from build123d import *

# Parameters (mm, degrees)
SKETCH_1_W      = 30
SKETCH_1_H      = 2
EXTRUDE_2_DEPTH = 2


with BuildPart() as part:
    # 草图1 → 凸台-拉伸2 (new body)
    with BuildSketch(Plane.XY):
        Polygon((-8, 49), (-8, 45), (2, 45), (2, 33.89311496), (2, -33.9722289), (2, -44.34252785), (-8, -44.34252785), (-8, -48.34252785), (-10, -48.34252785), (-10, -68.34252785), (-8, -68.34252785), (-8, -88.34252785), (-10, -88.34252785), (-10, -108.34252785), (-8, -108.34252785), (-8, -128.34252785), (-10, -128.34252785), (-10, -144), (-8, -144), (27, -144), (29, -144), (29, -128.34252785), (27, -128.34252785), (27, -108.34252785), (29, -108.34252785), (29, -88.34252785), (27, -88.34252785), (27, -68.34252785), (29, -68.34252785), (29, -48.34252785), (27, -48.34252785), (27, -28.34252785), (29, -28.34252785), (29, -8.34252785), (27, -8.34252785), (27, 11.65747215), (29, 11.65747215), (29, 31.65747215), (27, 31.65747215), (27, 51.65747215), (29, 51.65747215), (29, 59), (-10, 59), (-10, 49), align=None)
        Polygon((9.5, -54.22154055), (24.5, -54.22154055), (24.5, -56.22154055), (-5.5, -56.22154055), (-5.5, -54.22154055), align=None, mode=Mode.SUBTRACT)
        with Locations((9.5, -95.22154055)):
            Rectangle(SKETCH_1_W, SKETCH_1_H, mode=Mode.SUBTRACT)
        with Locations((9.5, -135.22154055)):
            Rectangle(SKETCH_1_W, SKETCH_1_H, mode=Mode.SUBTRACT)
    extrude(amount=EXTRUDE_2_DEPTH)


solid = part.part
For this review, take the finished solid that the model builds, in its own axes (mm). Give positions to 0.01 mm unless a question says otherwise; leave off trailing zeros. Loops run counter-clockwise (first coordinate to the right, second up) from the corner with the lowest first, then second, coordinate; pieces in that order, holes last.
Item 1: Take a section at C-C, the plane z = 1.1. Give the number of separate pieces and of enclosed holes in the cut face, and give its area (3 significant figures).
Item 2: Take a section at A-A, the plane x = 10. State the section outline as (y, z) points.
Item 3: Take a section at D-D, the plane y = 39. State the section outline as (x, z) points.
Item 4: Draft analysis for pull direction Z (two halves, no side actions). For faces 1 (the flat face through (14, -41, 0)), 2 (the flat face through (14, -41, 2)), state which applies: +Z half, -Z half, draft (parallel to the pull), parting line (faces both ways), or undercut.
Item 5: Insertion check: pin 1 (0.6 mm diameter, centred on y = -36, z = 0.5, fed in from +X). The pin has a flat end and moves straight along its axis. Give the tip position at first contact, or say it passes through.
Item 6: For line 1 along Y through (x, z) = (9, 1.5); line 2 along Y through (x, z) = (-3, 1.55); line 3 along X through (y, z) = (-54.5, 1.7), list the stretches that pass through material, from the lowest coordinate up.
Item 7: Take a section at B-B, the plane x = -0.5. State the section outline as (y, z) points.
Calculated:
1. separate pieces: 1
1. enclosed holes: 3
1. area: 6,370 mm2
2. outline: (-144, 0) - (-136.22, 0) - (-136.22, 2) - (-144, 2) - close; (-134.22, 0) - (-96.22, 0) - (-96.22, 2) - (-134.22, 2) - close; (-94.22, 0) - (-56.22, 0) - (-56.22, 2) - (-94.22, 2) - close; (-54.22, 0) - (59, 0) - (59, 2) - (-54.22, 2) - close
3. outline: (2, 0) - (27, 0) - (27, 2) - (2, 2) - close
4. face 1: -Z half
4. face 2: +Z half
5. pin 1: stops at x = 27
6. line 1: y = -144 to -136.22, -134.22 to -96.22, -94.22 to -56.22, -54.22 to 59
6. line 2: y = -144 to -136.22, -134.22 to -96.22, -94.22 to -56.22, -54.22 to -44.34, 45 to 59
6. line 3: x = -10 to -5.5, 24.5 to 29
7. outline: (-144, 0) - (-136.22, 0) - (-136.22, 2) - (-144, 2) - close; (-134.22, 0) - (-96.22, 0) - (-96.22, 2) - (-134.22, 2) - close; (-94.22, 0) - (-56.22, 0) - (-56.22, 2) - (-94.22, 2) - close; (-54.22, 0) - (-44.34, 0) - (-44.34, 2) - (-54.22, 2) - close; (45, 0) - (59, 0) - (59, 2) - (45, 2) - close
